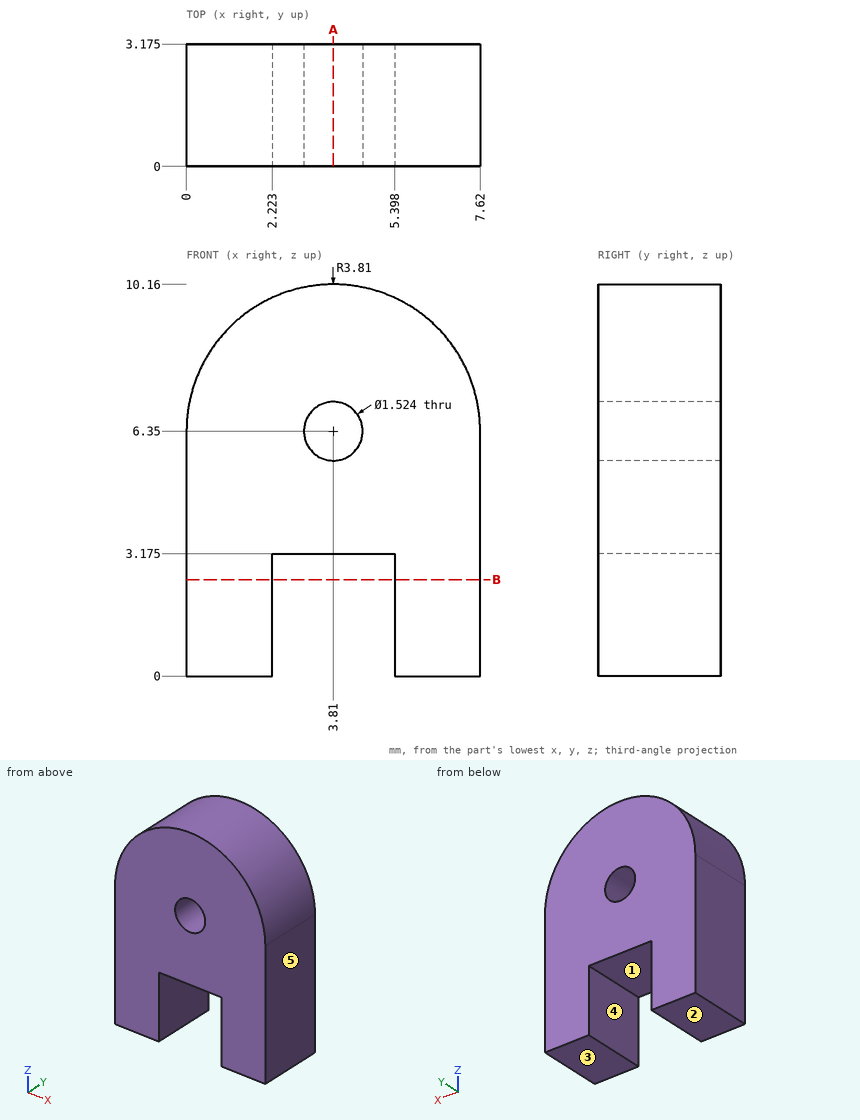
Check sheet for the drawn part. Datum: minimum x, y, z corner. Units: mm. A direction names the side the tool comes from. Give positions to 0.01 mm unless a question says otherwise; leave off trailing zeros. Order: outer loops, then holes, each group sorted by start corner. A loop starts at its lowest first (then second) coordinate and runs counter-clockwise, first axis right, second up. Notation, with made-up numbers: (-13.75, 49.25) - (16.25, 49.25) arc R20 cw to (16.25, 55.25) - close; hole circle Ø10 at (16, -17.75). An arc over 180 degrees is marked (long way). Answer as a JSON object with one key per item and string values.
(1) Cross-section at B-B (z = 2.5). Record the cut outline in (x, y) (1 decimal).
Report:
{"outline": "(0, 0) - (2.2, 0) - (2.2, 3.2) - (0, 3.2) - close; (5.4, 0) - (7.6, 0) - (7.6, 3.2) - (5.4, 3.2) - close"}
(2) Tool access check on the marked faces 1 and 2. Record the directions out of +Z, -Z, +X, -X, +Y, -Y that give a thin tool (end or side, any length) a straight path to the whole face; none if there is none.
Report:
{"face 1": "-Z, +Y, -Y", "face 2": "-Z, +X, -X, +Y, -Y"}
(3) Cross-section at A-A (x = 3.81). Record the cut outline in (y, z) (1 decimal).
Report:
{"outline": "(0, 3.2) - (3.2, 3.2) - (3.2, 5.6) - (0, 5.6) - close; (0, 7.1) - (3.2, 7.1) - (3.2, 10.2) - (0, 10.2) - close"}
(4) Material ranges on line 1 (Z direction, x = 3.81, y = 0.85) (1 decimal); line 2 (X direction, y = 2, z = 1.25); line 3 (X direction, y = 2.45, z = 6.35), recorded low to high.
Report:
{"line 1": "3.2 to 5.6, 7.1 to 10.2", "line 2": "0 to 2.22, 5.4 to 7.62", "line 3": "0 to 3.05, 4.57 to 7.62"}
(5) Draft check along X on the marked faces 3, 4 and 5. Enter one of: released by +X, released by -X, zero draft, split by the parting line, or undercut.
Report:
{"face 3": "zero draft", "face 4": "undercut", "face 5": "released by +X"}
